Input: part model. Units: mm. Frame: model coordinates. Face numbers are marked on the shaded views. A direction names the side the tool comes from. Coordinates: 2 decimals unless noted, no trailing zeros. Loops run counter-clockwise (first coordinate to the right, second up) from the corner with the lowest first, then second, coordinate; pieces in that order, holes last.
```python
from build123d import *

# Parameters (mm, degrees)
SZKIC1_W                    = 104
SZKIC1_H                    = 64
DODANIE_WYCI_GNI_CIE1_DEPTH = 2
SZKIC2_W                    = 8
SZKIC2_H                    = 8
DODANIE_WYCI_GNI_CIE2_DEPTH = 20
SZKIC4_R                    = 1.6
DODANIE_WYCI_GNI_CIE3_DEPTH = 2
DODANIE_WYCI_GNI_CIE4_START = 2
SZKIC5_R                    = 1.6
DODANIE_WYCI_GNI_CIE4_DEPTH = 2
SFAZOWANIE1_SIZE            = 2
SZKIC6_W                    = 5.65685425
SZKIC6_H                    = 5.65685425
SZKIC6_R                    = 1.6
WYTNIJ_WYCI_GNI_CIE2_DEPTH  = 4
SZKIC6_AGAIN_R              = 1.6
WYTNIJ_WYCI_GNI_CIE3_DEPTH  = 6.2
DODANIE_WYCI_GNI_CIE5_DEPTH = 2
SZKIC8_W                    = 5.65685425
SZKIC8_H                    = 5.65685425
SZKIC8_R                    = 1.6
WYTNIJ_WYCI_GNI_CIE4_DEPTH  = 4
SZKIC8_2_R                  = 1.6
WYTNIJ_WYCI_GNI_CIE5_DEPTH  = 4.2
SZKIC8_3_W                  = 5.65685425
SZKIC8_3_H                  = 5.65685425
SZKIC8_3_R                  = 1.6
DODANIE_WYCI_GNI_CIE6_DEPTH = 2
WYTNIJ_WYCI_GNI_CIE6_START  = -4
SZKIC9_W                    = 5.65685425
SZKIC9_H                    = 5.65685425
SZKIC9_R                    = 1.6
WYTNIJ_WYCI_GNI_CIE6_DEPTH  = 4
WYTNIJ_WYCI_GNI_CIE7_START  = -4.2
SZKIC9_2_R                  = 1.6
WYTNIJ_WYCI_GNI_CIE7_DEPTH  = 4.2
DODANIE_WYCI_GNI_CIE7_START = -2
SZKIC9_3_W                  = 5.65685425
SZKIC9_3_H                  = 5.65685425
SZKIC9_3_R                  = 1.6
DODANIE_WYCI_GNI_CIE7_DEPTH = 2
SZKIC10_W                   = 20
SZKIC10_H                   = 10
SZKIC10_W_2                 = 27.5
SZKIC10_H_2                 = 19
WYTNIJ_WYCI_GNI_CIE8_DEPTH  = 9
SZKIC11_W                   = 2
SZKIC11_H                   = 2
DODANIE_WYCI_GNI_CIE8_DEPTH = 64
ZAOKR_GLENIE1_R             = 2


with BuildPart() as part:
    # Szkic1 → Dodanie-wyciągnięcie1 (new body)
    with BuildSketch(Plane(origin=(0, 0, 0), x_dir=(1, 0, 0), z_dir=(0, 1, 0))):
        with Locations((52, 32)):
            Rectangle(SZKIC1_W, SZKIC1_H)
    extrude(amount=DODANIE_WYCI_GNI_CIE1_DEPTH)

    # Szkic2 → Dodanie-wyciągnięcie2 (add)
    with BuildSketch(Plane(origin=(0, 2, 0), x_dir=(1, 0, 0), z_dir=(0, 1, 0))):
        with Locations((4, 60)):
            Rectangle(SZKIC2_W, SZKIC2_H)
        with Locations((4, 4)):
            Rectangle(SZKIC2_W, SZKIC2_H)
        with Locations((100, 4)):
            Rectangle(SZKIC2_W, SZKIC2_H)
        with Locations((100, 60)):
            Rectangle(SZKIC2_W, SZKIC2_H)
    extrude(amount=DODANIE_WYCI_GNI_CIE2_DEPTH)

    # Szkic4 → Dodanie-wyciągnięcie3 (add)
    # profile 1 of 2: a face of its own
    with BuildSketch(Plane.ZY):
        with BuildLine():
            Line((-8, 2), (-8, 22))
            Line((-8, 22), (-19.553012413, 22))
            ThreePointArc((-19.553012413, 22), (-32, 10.65), (-44.446987587, 22))
            Line((-44.446987587, 22), (-56, 22))
            Line((-56, 22), (-56, 2))
            Line((-56, 2), (-8, 2))
        make_face()
        with Locations((-47.5, 7.65)):
            Circle(SZKIC4_R, mode=Mode.SUBTRACT)
        with Locations((-16.5, 7.65)):
            Circle(SZKIC4_R, mode=Mode.SUBTRACT)
    # profile 2 of 2: a face of its own
    with BuildSketch(Plane.ZY):
        Polygon((-64, 22), (-64, 0), (0, 0), (0, 22), (-8, 22), (-8, 2), (-56, 2), (-56, 22), align=None)
    extrude(amount=DODANIE_WYCI_GNI_CIE3_DEPTH)

    # Szkic5 → Dodanie-wyciągnięcie4 (add)
    # profile 1 of 2: a face of its own
    with BuildSketch(Plane(origin=(104, 0, 0), x_dir=(0, 0, -1), z_dir=(1, 0, 0)).offset(DODANIE_WYCI_GNI_CIE4_START)):
        with BuildLine():
            Line((56, 2), (56, 22))
            Line((56, 22), (44.446987587, 22))
            ThreePointArc((44.446987587, 22), (32, 10.65), (19.553012413, 22))
            Line((19.553012413, 22), (8, 22))
            Line((8, 22), (8, 2))
            Line((8, 2), (56, 2))
        make_face()
        with Locations(Location((16.5, 7.65, 0), (0, 0, 180))):
            Circle(SZKIC5_R, mode=Mode.SUBTRACT)
        with Locations(Location((47.5, 7.65, 0), (0, 0, 180))):
            Circle(SZKIC5_R, mode=Mode.SUBTRACT)
    # profile 2 of 2: a face of its own
    with BuildSketch(Plane(origin=(104, 0, 0), x_dir=(0, 0, -1), z_dir=(1, 0, 0)).offset(DODANIE_WYCI_GNI_CIE4_START)):
        Polygon((0, 22), (0, 0), (64, 0), (64, 22), (56, 22), (56, 2), (8, 2), (8, 22), align=None)
    extrude(amount=-DODANIE_WYCI_GNI_CIE4_DEPTH)

    # Sfazowanie1
    sfazowanie1_edges = [part.edges().sort_by_distance(p)[0] for p in [
        (-2, 0, -32),
        (106, 0, -32),
    ]]
    chamfer(sfazowanie1_edges, length=SFAZOWANIE1_SIZE)

    # Szkic6 → Wytnij-wyciągnięcie2 (cut)
    # profile 1 of 4: a face of its own
    with BuildSketch(Plane.XZ):
        with Locations((4, -4)):
            Rectangle(SZKIC6_W, SZKIC6_H)
        with Locations(Location((4, -4, 0), (0, 0, 270))):
            Circle(SZKIC6_R, mode=Mode.SUBTRACT)
    # profile 2 of 4: a face of its own
    with BuildSketch(Plane.XZ):
        with Locations((4, -60)):
            Rectangle(SZKIC6_W, SZKIC6_H)
        with Locations(Location((4, -60, 0), (0, 0, 270))):
            Circle(SZKIC6_R, mode=Mode.SUBTRACT)
    # profile 3 of 4: a face of its own
    with BuildSketch(Plane.XZ):
        with Locations((100, -60)):
            Rectangle(SZKIC6_W, SZKIC6_H)
        with Locations(Location((100, -60, 0), (0, 0, 270))):
            Circle(SZKIC6_R, mode=Mode.SUBTRACT)
    # profile 4 of 4: a face of its own
    with BuildSketch(Plane.XZ):
        with Locations((100, -4)):
            Rectangle(SZKIC6_W, SZKIC6_H)
        with Locations(Location((100, -4, 0), (0, 0, 270))):
            Circle(SZKIC6_R, mode=Mode.SUBTRACT)
    extrude(amount=-WYTNIJ_WYCI_GNI_CIE2_DEPTH, mode=Mode.SUBTRACT)

    # Szkic6 again → Wytnij-wyciągnięcie3 (cut)
    with BuildSketch(Plane.XZ):
        with Locations(Location((4, -4, 0), (0, 0, 270))):
            Circle(SZKIC6_AGAIN_R)
        with Locations(Location((4, -60, 0), (0, 0, 270))):
            Circle(SZKIC6_AGAIN_R)
        with Locations(Location((100, -60, 0), (0, 0, 270))):
            Circle(SZKIC6_AGAIN_R)
        with Locations(Location((100, -4, 0), (0, 0, 270))):
            Circle(SZKIC6_AGAIN_R)
    extrude(amount=-WYTNIJ_WYCI_GNI_CIE3_DEPTH, mode=Mode.SUBTRACT)

    # Szkic6 → Dodanie-wyciągnięcie5 (add)
    # profile 1 of 4: a face of its own
    with BuildSketch(Plane.XZ):
        with Locations((4, -4)):
            Rectangle(SZKIC6_W, SZKIC6_H)
        with Locations(Location((4, -4, 0), (0, 0, 270))):
            Circle(SZKIC6_R, mode=Mode.SUBTRACT)
    # profile 2 of 4: a face of its own
    with BuildSketch(Plane.XZ):
        with Locations((4, -60)):
            Rectangle(SZKIC6_W, SZKIC6_H)
        with Locations(Location((4, -60, 0), (0, 0, 270))):
            Circle(SZKIC6_R, mode=Mode.SUBTRACT)
    # profile 3 of 4: a face of its own
    with BuildSketch(Plane.XZ):
        with Locations((100, -60)):
            Rectangle(SZKIC6_W, SZKIC6_H)
        with Locations(Location((100, -60, 0), (0, 0, 270))):
            Circle(SZKIC6_R, mode=Mode.SUBTRACT)
    # profile 4 of 4: a face of its own
    with BuildSketch(Plane.XZ):
        with Locations((100, -4)):
            Rectangle(SZKIC6_W, SZKIC6_H)
        with Locations(Location((100, -4, 0), (0, 0, 270))):
            Circle(SZKIC6_R, mode=Mode.SUBTRACT)
    extrude(amount=-DODANIE_WYCI_GNI_CIE5_DEPTH)

    # Szkic8 → Wytnij-wyciągnięcie4 (cut)
    # profile 1 of 2: a face of its own
    with BuildSketch(Plane(origin=(0, 0, -64), x_dir=(-1, 0, 0), z_dir=(0, 0, -1))):
        with Locations((-4, 12)):
            Rectangle(SZKIC8_W, SZKIC8_H)
        with Locations((-4, 12)):
            Circle(SZKIC8_R, mode=Mode.SUBTRACT)
    # profile 2 of 2: a face of its own
    with BuildSketch(Plane(origin=(0, 0, -64), x_dir=(-1, 0, 0), z_dir=(0, 0, -1))):
        with Locations((-100, 12)):
            Rectangle(SZKIC8_W, SZKIC8_H)
        with Locations((-100, 12)):
            Circle(SZKIC8_R, mode=Mode.SUBTRACT)
    extrude(amount=-WYTNIJ_WYCI_GNI_CIE4_DEPTH, mode=Mode.SUBTRACT)

    # Szkic8<2> → Wytnij-wyciągnięcie5 (cut)
    with BuildSketch(Plane(origin=(0, 0, -64), x_dir=(-1, 0, 0), z_dir=(0, 0, -1))):
        with Locations((-4, 12)):
            Circle(SZKIC8_2_R)
        with Locations((-100, 12)):
            Circle(SZKIC8_2_R)
    extrude(amount=-WYTNIJ_WYCI_GNI_CIE5_DEPTH, mode=Mode.SUBTRACT)

    # Szkic8<3> → Dodanie-wyciągnięcie6 (add)
    # profile 1 of 2: a face of its own
    with BuildSketch(Plane(origin=(0, 0, -64), x_dir=(-1, 0, 0), z_dir=(0, 0, -1))):
        with Locations((-4, 12)):
            Rectangle(SZKIC8_3_W, SZKIC8_3_H)
        with Locations((-4, 12)):
            Circle(SZKIC8_3_R, mode=Mode.SUBTRACT)
    # profile 2 of 2: a face of its own
    with BuildSketch(Plane(origin=(0, 0, -64), x_dir=(-1, 0, 0), z_dir=(0, 0, -1))):
        with Locations((-100, 12)):
            Rectangle(SZKIC8_3_W, SZKIC8_3_H)
        with Locations((-100, 12)):
            Circle(SZKIC8_3_R, mode=Mode.SUBTRACT)
    extrude(amount=-DODANIE_WYCI_GNI_CIE6_DEPTH)

    # Szkic9 → Wytnij-wyciągnięcie6 (cut)
    # profile 1 of 2: a face of its own
    with BuildSketch(Plane.XY.offset(WYTNIJ_WYCI_GNI_CIE6_START)):
        with Locations((100, 12)):
            Rectangle(SZKIC9_W, SZKIC9_H)
        with Locations(Location((100, 12, 0), (0, 0, 180))):
            Circle(SZKIC9_R, mode=Mode.SUBTRACT)
    # profile 2 of 2: a face of its own
    with BuildSketch(Plane.XY.offset(WYTNIJ_WYCI_GNI_CIE6_START)):
        with Locations((4, 12)):
            Rectangle(SZKIC9_W, SZKIC9_H)
        with Locations(Location((4, 12, 0), (0, 0, 180))):
            Circle(SZKIC9_R, mode=Mode.SUBTRACT)
    extrude(amount=WYTNIJ_WYCI_GNI_CIE6_DEPTH, mode=Mode.SUBTRACT)

    # Szkic9<2> → Wytnij-wyciągnięcie7 (cut)
    with BuildSketch(Plane.XY.offset(WYTNIJ_WYCI_GNI_CIE7_START)):
        with Locations(Location((100, 12, 0), (0, 0, 180))):
            Circle(SZKIC9_2_R)
        with Locations(Location((4, 12, 0), (0, 0, 180))):
            Circle(SZKIC9_2_R)
    extrude(amount=WYTNIJ_WYCI_GNI_CIE7_DEPTH, mode=Mode.SUBTRACT)

    # Szkic9<3> → Dodanie-wyciągnięcie7 (add)
    # profile 1 of 2: a face of its own
    with BuildSketch(Plane.XY.offset(DODANIE_WYCI_GNI_CIE7_START)):
        with Locations((100, 12)):
            Rectangle(SZKIC9_3_W, SZKIC9_3_H)
        with Locations(Location((100, 12, 0), (0, 0, 180))):
            Circle(SZKIC9_3_R, mode=Mode.SUBTRACT)
    # profile 2 of 2: a face of its own
    with BuildSketch(Plane.XY.offset(DODANIE_WYCI_GNI_CIE7_START)):
        with Locations((4, 12)):
            Rectangle(SZKIC9_3_W, SZKIC9_3_H)
        with Locations(Location((4, 12, 0), (0, 0, 180))):
            Circle(SZKIC9_3_R, mode=Mode.SUBTRACT)
    extrude(amount=DODANIE_WYCI_GNI_CIE7_DEPTH)

    # Szkic10 → Wytnij-wyciągnięcie8 (cut)
    with BuildSketch(Plane.XZ):
        with Locations((52, -32)):
            Rectangle(SZKIC10_W, SZKIC10_H)
        with Locations((28.25, -32)):
            Rectangle(SZKIC10_W_2, SZKIC10_H)
        with Locations((52, -17.5)):
            Rectangle(SZKIC10_W, SZKIC10_H_2)
        with Locations((52, -46.5)):
            Rectangle(SZKIC10_W, SZKIC10_H_2)
        with Locations((75.75, -32)):
            Rectangle(SZKIC10_W_2, SZKIC10_H)
    extrude(amount=-WYTNIJ_WYCI_GNI_CIE8_DEPTH, mode=Mode.SUBTRACT)

    # Szkic11 → Dodanie-wyciągnięcie8 (add)
    with BuildSketch(Plane.XY):
        with Locations((-1, 1)):
            Rectangle(SZKIC11_W, SZKIC11_H)
        with Locations((105, 1)):
            Rectangle(SZKIC11_W, SZKIC11_H)
    extrude(amount=-DODANIE_WYCI_GNI_CIE8_DEPTH)

    # Zaokrąglenie1
    zaokr_glenie1_edges = [part.edges().sort_by_distance(p)[0] for p in [
        (42, 1, -37),
        (14.5, 1, -37),
        (14.5, 1, -27),
        (42, 1, -27),
        (42, 1, -8),
        (62, 1, -8),
        (62, 1, -27),
        (89.5, 1, -27),
        (89.5, 1, -37),
        (62, 1, -37),
        (62, 1, -56),
        (42, 1, -56),
    ]]
    fillet(zaokr_glenie1_edges, radius=ZAOKR_GLENIE1_R)


solid = part.part
```
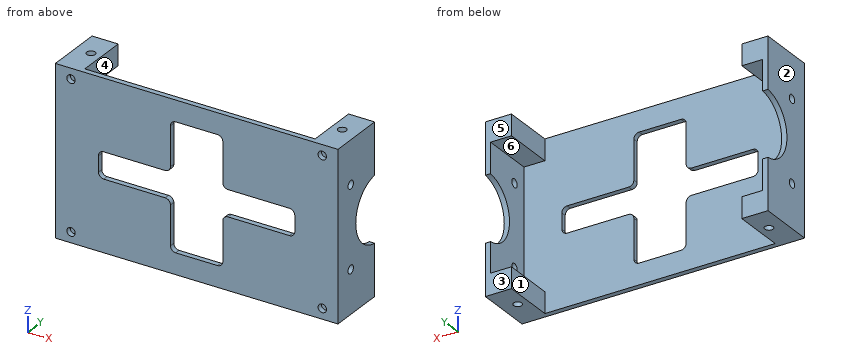
Item 1: Section query A-A (z = -47.5). Output: boundary loops of the cut face in (x, y).
Result:
outline: (-2, 0) - (42, 0) - (42, 2) - (0, 2) - (0, 6.05) - (-2, 6.05) - close; (-2, 9.25) - (0, 9.25) - (0, 22) - (-2, 22) - close; (62, 0) - (106, 0) - (106, 6.05) - (104, 6.05) - (104, 2) - (62, 2) - close; (104, 9.25) - (106, 9.25) - (106, 22) - (104, 22) - close
Item 2: Mould query, pull axis X, two halves, no side actions, for the marked faces 1, 2 and 3. Classes: +X half, -X half, draft (parallel to the pull), parting line (faces both ways), or undercut.
Result:
face 1: undercut
face 2: -X half
face 3: draft
Item 3: Section query B-B (y = 7.65). Count the separate pieces of the cut face and the enclosed holes in it, then the cut area to 3 significant figures.
Result:
separate pieces: 6
enclosed holes: 0
area: 486 mm2
Item 4: Contact query for flat-ended pins moving along their axis: P1, Ø1.7, axis at x = 101, y = 11.5, coming from the +Z side; P2, Ø2, axis at x = 29, z = -20, coming from the +Y side; P3, Ø2.5, axis at x = 100, y = 12, coming from the +Z side. Output: stop coordinate, or through.
Result:
P1: stops at z = 0
P2: stops at y = 2
P3: stops at z = -4.2
Item 5: Line query: L1, parallel to Y at x = 100, z = -1.6; L2, parallel to X at y = 12, z = -1.45; L3, parallel to X at y = 14.25, z = -55.5. Output: solid intervals per line, ascending.
Result:
L1: y = 0 to 2, 4 to 10.4, 13.6 to 22
L2: x = -2 to 2.4, 5.6 to 8, 96 to 98.4, 101.6 to 106
L3: x = -2 to 0, 104 to 106
Item 6: Reachability of the marked faces 4, 5 and 6 from +Z, -Z, +X, -X, +Y, -Y: full face, straight path, thin tool, end or side. Return the list, or none.
Result:
face 4: +Z, -Z, +Y
face 5: +Z, -Z, +X, -X, +Y
face 6: +Y
Item 7: Section query D-D (y = 20). Output: boundary loops of the cut face in (x, z), then the cut area to 3 significant figures.
Result:
outline: (-2, -64) - (8, -64) - (8, -56) - (0, -56) - (0, -44.1) - (-2, -44.1) - close; (-2, -19.9) - (0, -19.9) - (0, -8) - (8, -8) - (8, 0) - (-2, 0) - close; (96, -64) - (106, -64) - (106, -44.1) - (104, -44.1) - (104, -56) - (96, -56) - close; (96, -8) - (104, -8) - (104, -19.9) - (106, -19.9) - (106, 0) - (96, 0) - close
area: 415 mm2
Item 8: Section query C-C (z = -32). Output: boundary loops of the cut face in (x, y).
Result:
outline: (-2, 0) - (14.5, 0) - (14.5, 2) - (0, 2) - (0, 10.65) - (-2, 10.65) - close; (89.5, 0) - (106, 0) - (106, 10.65) - (104, 10.65) - (104, 2) - (89.5, 2) - close
